Can you work these out from the drawing? Everything is in mm from the part's minimum corner. A direction names the side the tool comes from. Round coordinates to 2 decimals unless told otherwise and drop trailing zeros. Loops run counter-clockwise (first coordinate to the right, second up) from the corner with the lowest first, then second, coordinate; pieces in that order, holes last. Notation, with made-up numbers: M 81,-5 L 130,-5 A18 ccw 130,11 Z; hole C -5,84 d2. An arc over 180 degrees is marked long. Use a Markdown table: item, result.
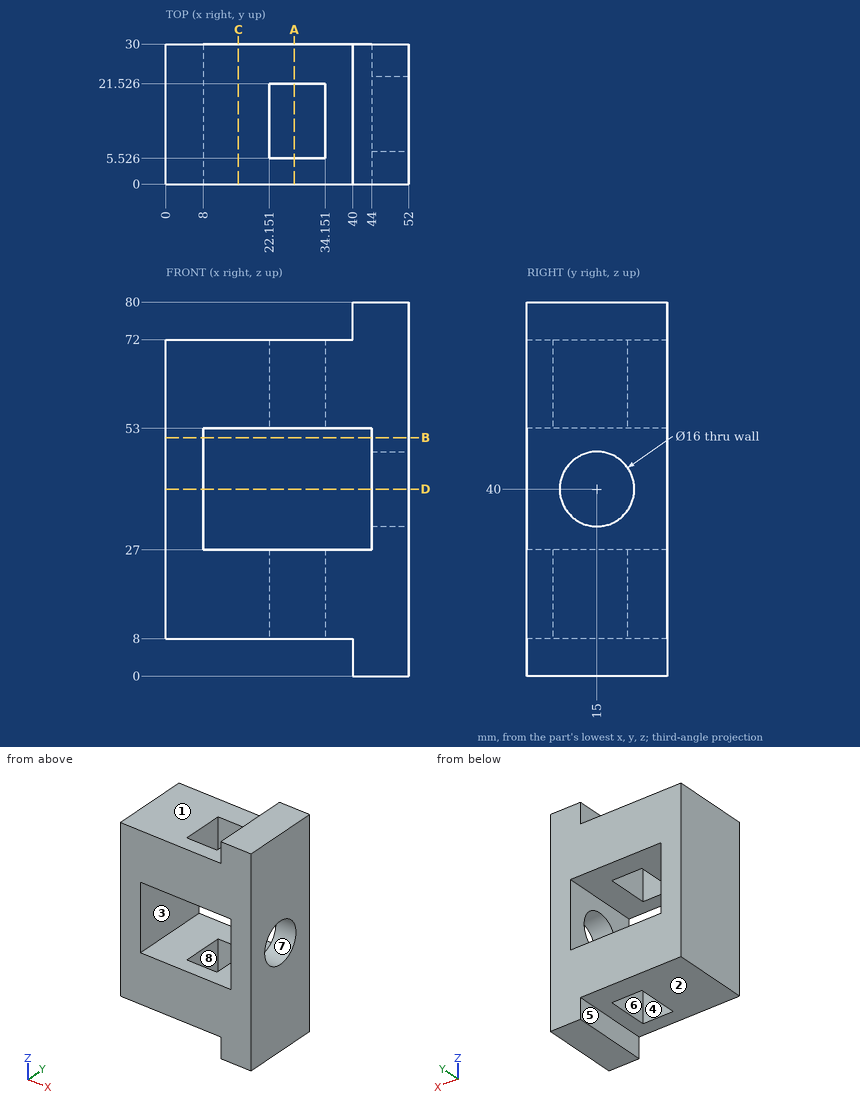
1. We'd pull the mould along X, two halves only. Please class the marked faces 5, 6, 7 and 8: +X half, -X half, draft (parallel to the pull), parting line (faces both ways), or undercut.
Answer sheet:
| item | result |
|---|---|
| face 5 | -X half |
| face 6 | undercut |
| face 7 | draft |
| face 8 | undercut |
2. For pin 1 Ø9 at (x, y) = (25, 10) entering from +Z; pin 2 Ø4 at (y, z) = (16.5, 5.5) entering from -X, each with a flat end and sliding along its axis, tell me the tip position at first contact or that it passes through.
Answer sheet:
| item | result |
|---|---|
| pin 1 | z = 72 |
| pin 2 | x = 40 |
3. Imagine slicing it at A-A, the plane x = 27.5. Write out the boundary of the cut face in (y, z).
Answer sheet:
| item | result |
|---|---|
| outline | M 0,8 L 5.53,8 L 5.53,27 L 0,27 Z; M 0,53 L 5.53,53 L 5.53,72 L 0,72 Z; M 21.53,8 L 30,8 L 30,27 L 21.53,27 Z; M 21.53,53 L 30,53 L 30,72 L 21.53,72 Z |
4. Imagine slicing it at D-D, the plane z = 40. Write out the boundary of the cut face in (x, y).
Answer sheet:
| item | result |
|---|---|
| outline | M 0,0 L 8,0 L 8,30 L 0,30 Z; M 44,0 L 52,0 L 52,7 L 44,7 Z; M 44,23 L 52,23 L 52,30 L 44,30 Z |
5. Which directions (+Z, -Z, +X, -X, +Y, -Y) give clear straight access to the entire face, cutting with the end or side of a thin tool? Please do the marked faces 1, 2, 3 and 4.
Answer sheet:
| item | result |
|---|---|
| face 1 | +Z, -X, +Y, -Y |
| face 2 | -Z, -X, +Y, -Y |
| face 3 | +Y, -Y |
| face 4 | +Z, -Z |
6. Imagine slicing it at B-B, the plane z = 51. Write out the boundary of the cut face in (x, y), then the cut area to 3 significant figures.
Answer sheet:
| item | result |
|---|---|
| outline | M 0,0 L 8,0 L 8,30 L 0,30 Z; M 44,0 L 52,0 L 52,30 L 44,30 Z |
| area | 480 mm2 |
7. I need wall thicknesses on probe 1 along Z at (x, y) = (46.5, 15); probe 2 along Z at (x, y) = (10, 24.25); probe 3 along X at (y, z) = (6.75, 37.5). Which ranges of each line are inside material? Lowest first, please. Write a range as from..to.
Answer sheet:
| item | result |
|---|---|
| probe 1 | 0..32, 48..80 |
| probe 2 | 8..27, 53..72 |
| probe 3 | 0..8, 44..52 |
8. Imagine slicing it at C-C, the plane x = 15.5. Write out the boundary of the cut face in (y, z).
Answer sheet:
| item | result |
|---|---|
| outline | M 0,8 L 30,8 L 30,27 L 0,27 Z; M 0,53 L 30,53 L 30,72 L 0,72 Z |
